For this review, take the finished solid that the model builds, in its own axes (mm). Face numbers are marked on the shaded views. Give positions to 0.01 mm unless a question says otherwise; leave off trailing zeros. Answer as CSV lines item,"result". Start each with the question number.
1. Mouldability with a two-part tool opening along Z and no side actions: class the marked faces 1, 2 and 3 as pulls with the +Z half, pulls with the -Z half, needs draft (parallel to the pull), parting line crosses it, or undercut.
2. Clearance check with flat-ended pins moving along their axes: P1, Ø10, axis at x = 22.5, y = 11, coming from the -Z side; P2, Ø3, axis at x = 22.5, z = -1.5, coming from the +Y side; P3, Ø6, axis at x = 23, z = 12, coming from the -Y side; P4, Ø17, axis at y = -3.5, z = -5, coming from the +X side (3 decimals). State where each tip first meets the part, or that it passes through.
3. For line 1 along Y through (x, z) = (19.5, 0); line 2 along Z through (x, y) = (17.5, 0); line 3 along X through (y, z) = (14, -2) (3 decimals), list the stretches that pass through material, from the lowest coordinate up.
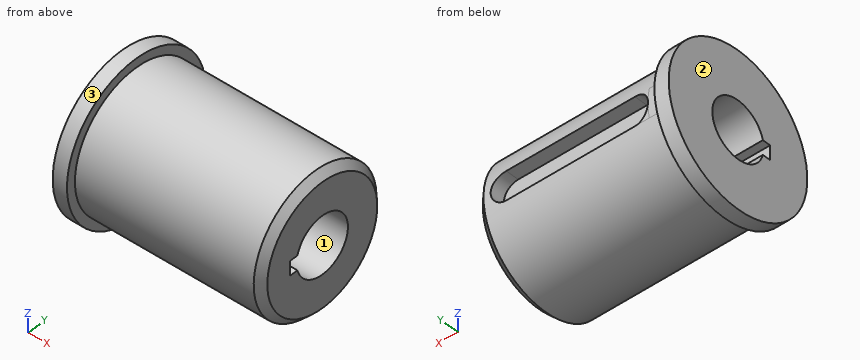
from build123d import *

# Parameters (mm, degrees)
SKETCH1_R           = 15.1892
SKETCH1_R_2         = 6.35
BOSS_EXTRUDE1_DEPTH = 41.275
SKETCH2_W           = 3.175
SKETCH2_H           = 3.175
SKETCH2_W_2         = 6.35
SKETCH2_H_2         = 6.35
CUT_EXTRUDE1_DEPTH  = 47.530089
BOSS_EXTRUDE2_START = 3.175
SKETCH3_R           = 17.145
BOSS_EXTRUDE2_DEPTH = 3.175
BOSS_EXTRUDE3_DEPTH = 3.175
BOSS_EXTRUDE4_START = -3.175
SKETCH5_R           = 15.1892
SKETCH5_R_2         = 10.967899
BOSS_EXTRUDE4_DEPTH = 3.175
FILLET1_R           = 3.175
CHAMFER1_SIZE       = 1.5875


with BuildPart() as part:
    # Sketch1 → Boss-Extrude1 (new body)
    with BuildSketch(Plane(origin=(0, 0, 0), x_dir=(0, 0, -1), z_dir=(1, 0, 0))):
        Circle(SKETCH1_R)
        Circle(SKETCH1_R_2, mode=Mode.SUBTRACT)
    extrude(amount=BOSS_EXTRUDE1_DEPTH)

    # Sketch2 → Cut-Extrude1 (cut, through all)
    with BuildSketch(Plane(origin=(41.275, 0, 0), x_dir=(0, 0, -1), z_dir=(1, 0, 0))):
        with Locations((0, -6.35)):
            Rectangle(SKETCH2_W, SKETCH2_H)
        with Locations((0, 15.08125)):
            Rectangle(SKETCH2_W_2, SKETCH2_H_2)
    extrude(amount=-CUT_EXTRUDE1_DEPTH, mode=Mode.SUBTRACT)

    # Sketch3 → Boss-Extrude2 (add)
    # profile 1 of 2: a face of its own
    with BuildSketch(Plane.ZY.offset(BOSS_EXTRUDE2_START)):
        Circle(SKETCH3_R)
        with BuildLine():
            Line((-3.175, 11.90625), (3.175, 11.90625))
            Line((3.175, 11.90625), (3.175, 14.853659))
            ThreePointArc((3.175, 14.853659), (0, -15.1892), (-3.175, 14.853659))
            Line((-3.175, 14.853659), (-3.175, 11.90625))
        make_face(mode=Mode.SUBTRACT)
    # profile 2 of 2: a face of its own
    with BuildSketch(Plane.ZY.offset(BOSS_EXTRUDE2_START)):
        with BuildLine():
            Line((3.175, 14.853659), (3.175, 11.90625))
            Line((3.175, 11.90625), (-3.175, 11.90625))
            Line((-3.175, 11.90625), (-3.175, 14.853659))
            ThreePointArc((-3.175, 14.853659), (0, -15.1892), (3.175, 14.853659))
        make_face()
        with BuildLine():
            Line((-1.5875, -7.9375), (-1.5875, -6.148361))
            ThreePointArc((-1.5875, -6.148361), (0, 6.35), (1.5875, -6.148361))
            Line((1.5875, -6.148361), (1.5875, -7.9375))
            Line((1.5875, -7.9375), (-1.5875, -7.9375))
        make_face(mode=Mode.SUBTRACT)
    extrude(amount=-BOSS_EXTRUDE2_DEPTH)

    # Sketch4 → Boss-Extrude3 (add)
    with BuildSketch(Plane(origin=(0, 0, 0), x_dir=(0, 0, -1), z_dir=(1, 0, 0))):
        with BuildLine():
            ThreePointArc((3.175, 14.853659), (0, 15.1892), (-3.175, 14.853659))
            Line((-3.175, 14.853659), (-3.175, 11.90625))
            Line((-3.175, 11.90625), (3.175, 11.90625))
            Line((3.175, 11.90625), (3.175, 14.827684))
            Line((3.175, 14.827684), (3.175, 14.853659))
        make_face()
    extrude(amount=BOSS_EXTRUDE3_DEPTH)

    # Sketch5 → Boss-Extrude4 (add)
    with BuildSketch(Plane(origin=(41.275, 0, 0), x_dir=(0, 0, -1), z_dir=(1, 0, 0)).offset(BOSS_EXTRUDE4_START)):
        Circle(SKETCH5_R)
        Circle(SKETCH5_R_2, mode=Mode.SUBTRACT)
    extrude(amount=BOSS_EXTRUDE4_DEPTH)

    # Fillet1
    # the kernel refuses this fillet: 3.175 mm, written as the material it adds along each edge
    with BuildSketch(Plane(origin=(3.175, 22.791159, -3.175), x_dir=(1, 0, 0), z_dir=(0, -1, 0))) as fillet1_piece_1_section:
        with BuildLine():
            CenterArc((FILLET1_R, FILLET1_R), FILLET1_R, 180, 90)
            Line((0, FILLET1_R), (0, 0))
            Line((0, 0), (FILLET1_R, 0))
        make_face()
    fillet1_piece_1 = extrude(amount=10.884909, mode=Mode.PRIVATE)
    fillet1_piece_1 = fillet1_piece_1 & Plane(origin=(3.873842, 0, 0), x_dir=(0, 0, -1), z_dir=(-1, 0, 0)) * Cylinder(15.1892, 35, mode=Mode.PRIVATE)
    add(fillet1_piece_1)
    with BuildSketch(Plane(origin=(3.175, 22.791159, 3.175), x_dir=(1, 0, 0), z_dir=(0, -1, 0))) as fillet1_piece_2_section:
        with BuildLine():
            CenterArc((FILLET1_R, -FILLET1_R), FILLET1_R, 90, 90)
            Line((0, -FILLET1_R), (0, 0))
            Line((0, 0), (FILLET1_R, 0))
        make_face()
    fillet1_piece_2 = extrude(amount=10.884909, mode=Mode.PRIVATE)
    fillet1_piece_2 = fillet1_piece_2 & Plane(origin=(3.873846, 0, 0), x_dir=(0, 0, -1), z_dir=(-1, 0, 0)) * Cylinder(15.1892, 35, mode=Mode.PRIVATE)
    add(fillet1_piece_2)
    with BuildSketch(Plane(origin=(38.1, 11.90625, 3.175), x_dir=(0, 0, -1), z_dir=(0, 1, 0))) as fillet1_piece_3_section:
        with BuildLine():
            CenterArc((FILLET1_R, FILLET1_R), FILLET1_R, 180, 90)
            Line((0, FILLET1_R), (0, 0))
            Line((0, 0), (FILLET1_R, 0))
        make_face()
    fillet1_piece_3 = extrude(amount=10.884909, mode=Mode.PRIVATE)
    fillet1_piece_3 = fillet1_piece_3 & Plane(origin=(37.401164, 0, 0), x_dir=(0, 0, -1), z_dir=(-1, 0, 0)) * Cylinder(15.1892, 35, mode=Mode.PRIVATE)
    add(fillet1_piece_3)
    with BuildSketch(Plane(origin=(38.1, 22.791159, -3.175), x_dir=(-1, 0, 0), z_dir=(0, -1, 0))) as fillet1_piece_4_section:
        with BuildLine():
            CenterArc((FILLET1_R, -FILLET1_R), FILLET1_R, 90, 90)
            Line((0, -FILLET1_R), (0, 0))
            Line((0, 0), (FILLET1_R, 0))
        make_face()
    fillet1_piece_4 = extrude(amount=10.884909, mode=Mode.PRIVATE)
    fillet1_piece_4 = fillet1_piece_4 & Plane(origin=(37.401158, 0, 0), x_dir=(0, 0, -1), z_dir=(-1, 0, 0)) * Cylinder(15.1892, 35, mode=Mode.PRIVATE)
    add(fillet1_piece_4)

    # Chamfer1
    chamfer1_edges = [part.edges().sort_by_distance(p)[0] for p in [
        (41.275, -14.853659, 3.175),
    ]]
    chamfer(chamfer1_edges, length=CHAMFER1_SIZE)


solid = part.part
Result set:
1,face 1,"undercut"
1,face 2,"needs draft"
1,face 3,"parting line crosses it"
2,P1,"z = -13.95"
2,P2,"y = 11.91"
2,P3,"y = -12.24"
2,P4,"x = 41.275"
3,line 1,"-15.19 to -7.94, 6.35 to 11.91"
3,line 2,"-15.19 to -6.35, 6.35 to 15.19"
3,line 3,"-3.175 to 3.884, 37.391 to 40.735"
